```python
from build123d import *

# Parameters (mm, degrees)
EXTRUDE_1_DEPTH     = 23
CUT_EXTRUDE_3_DEPTH = 20
SKETCH_3_R          = 1.3
CUT_EXTRUDE_4_DEPTH = 4
SKETCH_4_W          = 42.5
SKETCH_4_H          = 6.002604642
CUT_EXTRUDE_5_DEPTH = 10


with BuildPart() as part:
    # Эскиз1 → Бобышка-Вытянуть1 (new body)
    with BuildSketch(Plane(origin=(0, 0, 0), x_dir=(1, 0, 0), z_dir=(0, 1, 0))):
        Polygon((0, 0), (-42.5, 0), (-58.75, 0), (-58.75, 3.3), (-42.5, 3.3), (-42.5, 20.3), (-33.5, 20.3), (-33.5, 3.3), (-9, 3.3), (-9, 20.3), (0, 20.3), (0, 3.3), (16.25, 3.3), (16.25, 0), align=None)
    extrude(amount=EXTRUDE_1_DEPTH)

    # Эскиз2 → Вырез-Вытянуть3 (cut)
    with BuildSketch(Plane.XZ):
        with BuildLine():
            Line((-9, -3.3), (-9, -20.3))
            ThreePointArc((-9, -20.3), (-4.5, -15.8), (0, -20.3))
            Line((0, -20.3), (0, -3.3))
            Line((0, -3.3), (-9, -3.3))
        make_face()
        with BuildLine():
            Line((-33.5, -3.3), (-42.5, -3.3))
            Line((-42.5, -3.3), (-42.5, -20.3))
            ThreePointArc((-42.5, -20.3), (-38, -15.8), (-33.5, -20.3))
            Line((-33.5, -20.3), (-33.5, -3.3))
        make_face()
    extrude(amount=-CUT_EXTRUDE_3_DEPTH, mode=Mode.SUBTRACT)

    # Эскиз3 → Вырез-Вытянуть4 (cut)
    with BuildSketch(Plane.XY):
        with Locations((-31.25, 2)):
            Circle(SKETCH_3_R)
        with Locations((-11.41399061, 2)):
            Circle(SKETCH_3_R)
    extrude(amount=-CUT_EXTRUDE_4_DEPTH, mode=Mode.SUBTRACT)

    # Эскиз4 → Вырез-Вытянуть5 (cut)
    with BuildSketch(Plane.XZ):
        with Locations((-21.25, -17.298697679)):
            Rectangle(SKETCH_4_W, SKETCH_4_H)
    extrude(amount=-CUT_EXTRUDE_5_DEPTH, mode=Mode.SUBTRACT)


solid = part.part
```
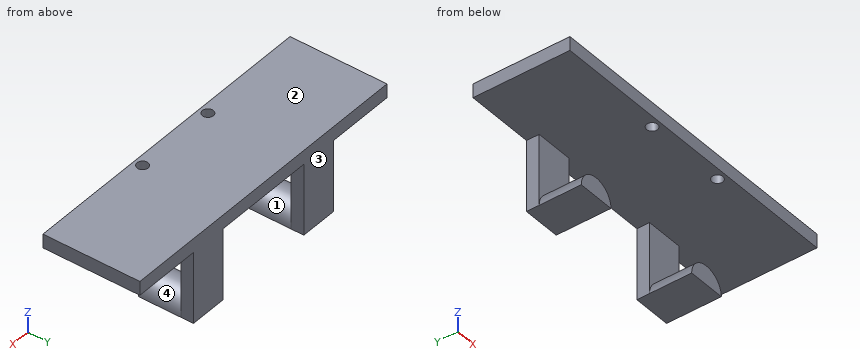
Could you check a few things on this model? Use its own coordinates, in mm. Face numbers are marked on the shaded views. A direction names the side the tool comes from. Round coordinates to 2 decimals unless told otherwise and drop trailing zeros. Loops run counter-clockwise (first coordinate to the right, second up) from the corner with the lowest first, then second, coordinate; pieces in that order, holes last. Notation, with made-up numbers: (-32.75, 88.5) -> (-8.75, 88.5) arc R8 cw to (-8.75, 93.5) -> close; hole circle Ø11 at (-2, 54.5). An arc over 180 degrees is marked (long way). Put each result on its own line as item: value.
Q1. Which directions (+Z, -Z, +X, -X, +Y, -Y) give clear straight access to the entire face, cutting with the end or side of a thin tool? Please do the marked faces 1 and 2.
Checks:
face 1: -Y
face 2: +Z, +X, -X, +Y, -Y
Q2. I want a section at B-B on x = -31.25. Write out the boundary of the cut face in (y, z).
Checks:
outline: (0, -3.3) -> (0.7, -3.3) -> (0.7, 0) -> (0, 0) -> close; (3.3, -3.3) -> (23, -3.3) -> (23, 0) -> (3.3, 0) -> close
Q3. I want a section at C-C on y = 2. Write out the boundary of the cut face in (x, z).
Checks:
outline: (-58.75, -3.3) -> (-32.55, -3.3) -> (-32.55, 0) -> (-58.75, 0) -> close; (-29.95, -3.3) -> (-12.71, -3.3) -> (-12.71, 0) -> (-29.95, 0) -> close; (-10.11, -3.3) -> (16.25, -3.3) -> (16.25, 0) -> (-10.11, 0) -> close
Q4. For pin 1 Ø8 at (x, y) = (-26.5, 17.5) entering from -Z; pin 2 Ø10 at (x, z) = (-4.5, -15) entering from -Y; pin 3 Ø0.9 at (y, z) = (22, -10) entering from -X, each with a flat end and sliding along its axis, tell me the tip position at first contact or that it passes through.
Checks:
pin 1: z = -3.3
pin 2: y = 10
pin 3: x = -42.5
Q5. Thinking about a two-plate mould opening in X: for the marked faces 3 and 4, which applies, pulls with the +X half, pulls with the -X half, needs draft (parallel to the pull), parting line crosses it, or undercut?
Checks:
face 3: needs draft
face 4: undercut
Q6. I want a section at D-D on y = 5. Write out the boundary of the cut face in (x, z).
Checks:
outline: (-58.75, -3.3) -> (16.25, -3.3) -> (16.25, 0) -> (-58.75, 0) -> close
Q7. I want a section at A-A on z = -8.5. Write out the boundary of the cut face in (x, y).
Checks:
outline: (-42.5, 20) -> (-33.5, 20) -> (-33.5, 23) -> (-42.5, 23) -> close; (-9, 20) -> (0, 20) -> (0, 23) -> (-9, 23) -> close
Q8. Please list where these lines run through material, in increasing order: line 1 (Y direction, x = -31.25, z = -2.5); line 2 (Z direction, x = -27, y = 16); line 3 (Y direction, x = -36.5, z = -8.5). Write a range as from..to.
Checks:
line 1: 0..0.7, 3.3..23
line 2: -3.3..0
line 3: 20..23
